from build123d import *

# Parameters (mm, degrees)
RESSALTO_EXTRUS_O1_DEPTH   = 30
CORTE_EXTRUS_O1_DEPTH      = 117.431310222
CORTE_EXTRUS_O1_DEPTH_BACK = 117.431310222
ESBO_O3_W                  = 24
ESBO_O3_H                  = 60
ESBO_O4_W                  = 122.227571884
ESBO_O4_H                  = 20
CORTE_EXTRUS_O3_DEPTH      = 20
ESBO_O6_W                  = 80
ESBO_O6_H                  = 31
CORTE_EXTRUS_O5_DEPTH      = 15
ESBO_O8_W                  = 48.18
ESBO_O8_H                  = 13.200484169
CORTE_EXTRUS_O6_DEPTH      = 15
ESBO_O9_W                  = 75
ESBO_O9_H                  = 48
CORTE_EXTRUS_O7_DEPTH      = 20
ESBO_O10_W                 = 48.7
ESBO_O10_H                 = 6.666237126
CORTE_EXTRUS_O8_DEPTH      = 15


with BuildPart() as part:
    # Esboço2 → Ressalto-extrusão1 (new body)
    with BuildSketch(Plane(origin=(0, 0, 0), x_dir=(1, 0, 0), z_dir=(0, 1, 0))):
        Polygon((-45, -45), (45, -45), (67.5, -20), (67.5, 60), (45, 90), (-45, 90), (-67.5, 60), (-67.5, -20), align=None)
    extrude(amount=RESSALTO_EXTRUS_O1_DEPTH)

    # Esboço3 → Corte-extrusão1 (cut, two sides: drawn at the far end of the back side and taken through both)
    with BuildSketch(Plane(origin=(0, 30, 0), x_dir=(1, 0, 0), z_dir=(0, 1, 0)).offset(-CORTE_EXTRUS_O1_DEPTH_BACK)):
        with Locations((-55.5, 15.849651962)):
            Rectangle(ESBO_O3_W, ESBO_O3_H)
        with Locations((55.5, 15.849651962)):
            Rectangle(ESBO_O3_W, ESBO_O3_H)
    extrude(amount=CORTE_EXTRUS_O1_DEPTH + CORTE_EXTRUS_O1_DEPTH_BACK, mode=Mode.SUBTRACT)

    # Esboço4 → Corte-extrusão3 (cut)
    with BuildSketch(Plane(origin=(0, 30, 0), x_dir=(1, 0, 0), z_dir=(0, 1, 0))):
        with Locations((-2.959415656, 15.849651962)):
            Rectangle(ESBO_O4_W, ESBO_O4_H)
    extrude(amount=-CORTE_EXTRUS_O3_DEPTH, mode=Mode.SUBTRACT)

    # Esboço6 → Corte-extrusão5 (cut)
    with BuildSketch(Plane(origin=(0, 30, 0), x_dir=(1, 0, 0), z_dir=(0, 1, 0))):
        with Locations((0, -22.850832207)):
            Rectangle(ESBO_O6_W, ESBO_O6_H)
    extrude(amount=-CORTE_EXTRUS_O5_DEPTH, mode=Mode.SUBTRACT)

    # Esboço8 → Corte-extrusão6 (cut)
    with BuildSketch(Plane(origin=(0, 30, 0), x_dir=(1, 0, 0), z_dir=(0, 1, 0))):
        with Locations((0, -0.750590123)):
            Rectangle(ESBO_O8_W, ESBO_O8_H)
    extrude(amount=-CORTE_EXTRUS_O6_DEPTH, mode=Mode.SUBTRACT)

    # Esboço9 → Corte-extrusão7 (cut)
    with BuildSketch(Plane(origin=(0, 30, 0), x_dir=(1, 0, 0), z_dir=(0, 1, 0))):
        with Locations((0, 56.515889088)):
            Rectangle(ESBO_O9_W, ESBO_O9_H)
    extrude(amount=-CORTE_EXTRUS_O7_DEPTH, mode=Mode.SUBTRACT)

    # Esboço10 → Corte-extrusão8 (cut)
    with BuildSketch(Plane(origin=(0, 30, 0), x_dir=(1, 0, 0), z_dir=(0, 1, 0))):
        with Locations((0, 29.182770525)):
            Rectangle(ESBO_O10_W, ESBO_O10_H)
    extrude(amount=-CORTE_EXTRUS_O8_DEPTH, mode=Mode.SUBTRACT)


solid = part.part
Part model, mm, in its own coordinate system. A direction names the side the tool comes from. Coordinates: 2 decimals unless noted, no trailing zeros. Loops run counter-clockwise (first coordinate to the right, second up) from the corner with the lowest first, then second, coordinate; pieces in that order, holes last. Notation, with made-up numbers: M 68.25,45.5 L 100.25,45.5 A21 cw 100.25,74.5 Z; hole C -38,78 d8. An arc over 180 degrees is marked long. Use a Markdown table: item, result. Add a question column.
Q1. Mould opens along Z. For faces 3 (the flat face through (56.4, 14.8, -74.8)), 4 (the flat face through (43.5, 8, -15)), 5 (the flat face through (-1, 0, -23)) say: +Z half, -Z half, draft (parallel to the pull), parting line (faces both ways), or undercut.
Q2. Cut at A-A (x = 52). Write the cut outline in (y, z).
Q3. Probe L1, parallel to Z at x = 26.5, y = 14; L2, parallel to X at y = 18.75, z = -40.5; L3, parallel to Z at x = -16, y = 22.5. List the from-to ranges inside material, lowest first.
Q4. Cut at D-D (x = 35). Write the cut outline in (y, z), and give its area (4 significant figures).
Q5. Cut at C-C (y = 7.75). Write the cut outline in (x, z), and give its area (3 significant figures).
Q6. Pin check, flat tips, straight feed: P1, Ø7.5, axis at y = 25.5, z = 30, coming from the +X side (3 decimals); P2, Ø5.5, axis at x = 8, z = -28, coming from the +Y side; P3, Ø16, axis at x = 14.5, z = -15.5, coming from the +Y side; P4, Ø1.5, axis at y = 12, z = -16.5, coming from the -X side. Stop position of each tip, or through.
Q7. Which spindle directions (+Z, -Z, +X, -X, +Y, -Y) get a long thin tool onto all of the face, cutting with end or side? Do faces 1 (the flat face through (-56.1, 14.8, -75.2)), 2 (the flat face through (24.09, 23, 1)). Say none if no direction does.
Q8. Cut at B-B (z = -77). Write the cut outline in (x, y), and give its area (4 significant figures).
Worked out:
| question | item | result |
|---|---|---|
| 1 | face 3 | -Z half |
| 1 | face 4 | undercut |
| 1 | face 5 | draft |
| 2 | outline | M 0,-80.67 L 30,-80.67 L 30,-45.85 L 0,-45.85 Z; M 0,14.15 L 30,14.15 L 30,37.22 L 0,37.22 Z |
| 3 | L1 | z = -90 to -80.52, -32.52 to -25.85, -5.85 to 45 |
| 3 | L2 | x = -43.5 to -37.5, 37.5 to 43.5 |
| 3 | L3 | z = -90 to -80.52, 38.35 to 45 |
| 4 | outline | M 0,-90 L 30,-90 L 30,-80.52 L 10,-80.52 L 10,-32.52 L 30,-32.52 L 30,-25.85 L 10,-25.85 L 10,-5.85 L 30,-5.85 L 30,7.35 L 15,7.35 L 15,38.35 L 30,38.35 L 30,45 L 0,45 Z |
| 4 | area | 2,225 mm2 |
| 5 | outline | M -67.5,-60 L -45,-90 L 45,-90 L 67.5,-60 L 67.5,-45.85 L 43.5,-45.85 L 43.5,14.15 L 67.5,14.15 L 67.5,20 L 45,45 L -45,45 L -67.5,20 L -67.5,14.15 L -43.5,14.15 L -43.5,-45.85 L -67.5,-45.85 Z |
| 5 | area | 14,100 mm2 |
| 6 | P1 | stops at x = 61.875 |
| 6 | P2 | stops at y = 15 |
| 6 | P3 | stops at y = 10 |
| 6 | P4 | passes through |
| 7 | face 1 | -Z, -X, +Y, -Y |
| 7 | face 2 | +Y |
| 8 | outline | M -54.75,0 L 54.75,0 L 54.75,30 L 37.5,30 L 37.5,10 L -37.5,10 L -37.5,30 L -54.75,30 Z |
| 8 | area | 1,785 mm2 |
